Geometry: final body of the model. Coordinates: model frame, mm. A direction names the side the tool comes from. Coordinates: 2 decimals unless noted, no trailing zeros. Loops run counter-clockwise (first coordinate to the right, second up) from the corner with the lowest first, then second, coordinate; pieces in that order, holes last. Notation, with made-up numbers: (-31.5, 50.5) -> (-1.5, 50.5) arc R8 ccw to (-1.5, 60.5) -> close; hole circle Ø2 at (36, -16.75). An arc over 180 degrees is marked (long way). One line per item, written item: value. Start each with the question number.
from build123d import *

# Parameters (mm, degrees)
F0_W      = 30
F0_H      = 30
F1_DEPTH  = 30
F2_W      = 5.5
F2_H      = 5.5
F3_DEPTH  = 12
F4_W      = 5.5
F4_H      = 5.5
F5_DEPTH  = 12
F6_W      = 5.5
F6_H      = 5.5
F7_DEPTH  = 12
F8_W      = 5.5
F8_H      = 5.5
F9_DEPTH  = 12
F10_W     = 5.5
F10_H     = 5.5
F11_DEPTH = 12
F12_W     = 5.5
F12_H     = 5.5
F13_DEPTH = 12
F14_SIZE  = 10


with BuildPart() as f1:
    # F0 (on Top) → F1 (new body)
    with BuildSketch(Plane.XY):
        with Locations((15, -15)):
            Rectangle(F0_W, F0_H)
    extrude(amount=F1_DEPTH)

    # F2 (on face) → F3 (cut)
    with BuildSketch(Plane(origin=(0, 0, 0), x_dir=(0, -1, 0), z_dir=(-1, 0, 0))):
        with Locations((15, 15)):
            Rectangle(F2_W, F2_H)
    extrude(amount=-F3_DEPTH, mode=Mode.SUBTRACT)

    # F4 (on face) → F5 (cut)
    with BuildSketch(Plane.YZ.offset(30)):
        with Locations((-15, 15)):
            Rectangle(F4_W, F4_H)
    extrude(amount=-F5_DEPTH, mode=Mode.SUBTRACT)

    # F6 (on face) → F7 (cut)
    with BuildSketch(Plane(origin=(0, 0, 0), x_dir=(-1, 0, 0), z_dir=(0, 1, 0))):
        with Locations((-15, 15)):
            Rectangle(F6_W, F6_H)
    extrude(amount=-F7_DEPTH, mode=Mode.SUBTRACT)

    # F8 (on face) → F9 (cut)
    with BuildSketch(Plane(origin=(0, 0, 0), x_dir=(1, 0, 0), z_dir=(0, 0, -1))):
        with Locations((15, 15)):
            Rectangle(F8_W, F8_H)
    extrude(amount=-F9_DEPTH, mode=Mode.SUBTRACT)

    # F10 (on face) → F11 (cut)
    with BuildSketch(Plane.XY.offset(30)):
        with Locations((15, -15)):
            Rectangle(F10_W, F10_H)
    extrude(amount=-F11_DEPTH, mode=Mode.SUBTRACT)

    # F12 (on face) → F13 (cut)
    with BuildSketch(Plane.XZ.offset(30)):
        with Locations((15, 15)):
            Rectangle(F12_W, F12_H)
    extrude(amount=-F13_DEPTH, mode=Mode.SUBTRACT)

    # F14
    f14_edges = [f1.edges().sort_by_distance(p)[0] for p in [
        (15, -30, 0),
        (30, -30, 15),
        (15, -30, 30),
        (0, -30, 15),
        (30, -15, 0),
        (0, -15, 0),
        (15, 0, 0),
        (30, 0, 15),
        (30, -15, 30),
        (0, -15, 30),
        (15, 0, 30),
        (0, 0, 15),
    ]]
    chamfer(f14_edges, length=F14_SIZE)


solid = f1.part
1. Draft query along Y for faces 1 (the face through (5, -15, 5)), 2 (the face through (24, -12.25, 15)), 3 (the face through (25, -25, 15)). Return one class per face: released by +Y, released by -Y, zero draft, split by the parting line, or undercut.
2. Line query: L1, parallel to X at y = -13, z = 11; L2, parallel to X at y = -4.5, z = 14. Output: solid intervals per line, ascending. Write a range as [from, to].
3. Set-up query: faces 4 (the face through (12.25, -15, 6)), 5 (the face through (12, 0, 15)), 6 (the face through (15, -15, 18)), 7 (the face through (15, -6, 17.75)), 8 (the face through (15, -24, 17.75)). Return all of +Z, -Z, +X, -X, +Y, -Y with unobstructed straight access to the full face (end or side cutting, diameter ignored); none if empty.
4. Section A-A on x = 9. Return the cut outline in (y, z).
5. Section B-B on y = -4. Return the cut outline in (x, z), plus the area to 3 significant figures.
6. Pin query (flat end, axial travel): pin 1 Ø6 at (x, y) = (15.5, -13.5) entering from +Z; pin 2 Ø3 at (x, y) = (13.5, -26) entering from +Z; pin 3 Ø4 at (x, y) = (20.5, -8) entering from +Z; pin 4 Ø3 at (x, z) = (14.5, 16) entering from +Y. Return the tip coordinate at first contact, or that it passes through.
7. Section C-C on z = 15.25. Return the cut outline in (x, y), plus the area to 3 significant figures.
Checks:
1. face 1: zero draft
1. face 2: undercut
1. face 3: released by -Y
2. L1: [0, 12.25], [17.75, 30]
2. L2: [5.5, 12.25], [17.75, 24.5]
3. face 4: -Z
3. face 5: +Z, -Z, +X, -X, +Y
3. face 6: +Z
3. face 7: +Y
3. face 8: -Y
4. outline: (-29, 10) -> (-20, 1) -> (-10, 1) -> (-1, 10) -> (-1, 20) -> (-10, 29) -> (-20, 29) -> (-29, 20) -> close; hole (-17.75, 12.25) -> (-12.25, 12.25) -> (-12.25, 17.75) -> (-17.75, 17.75) -> close
5. outline: (6, 10) -> (10, 6) -> (20, 6) -> (24, 10) -> (24, 20) -> (20, 24) -> (10, 24) -> (6, 20) -> close; hole (12.25, 12.25) -> (17.75, 12.25) -> (17.75, 17.75) -> (12.25, 17.75) -> close
5. area: 262 mm²
6. pin 1: z = 30
6. pin 2: z = 25.5
6. pin 3: z = 29.94
6. pin 4: y = -12
7. outline: (0, -20) -> (10, -30) -> (12.25, -30) -> (12.25, -18) -> (17.75, -18) -> (17.75, -30) -> (20, -30) -> (30, -20) -> (30, -17.75) -> (18, -17.75) -> (18, -12.25) -> (30, -12.25) -> (30, -10) -> (20, 0) -> (17.75, 0) -> (17.75, -12) -> (12.25, -12) -> (12.25, 0) -> (10, 0) -> (0, -10) -> (0, -12.25) -> (12, -12.25) -> (12, -17.75) -> (0, -17.75) -> close
7. area: 436 mm²
